Could you check a few things on this model? Use its own coordinates, in mm. Coordinates: 2 decimals unless noted, no trailing zeros.
Autodesk Inventor part; units mm, degrees
ref_plane "Work Plane1" through (387.8168, 0.3965, 6.35) normal (0, 0, 1) x (1, 0, 0)
ref_plane "YZ Plane" through (0, 0, 0) normal (1, 0, 0) x (0, 1, 0)
ref_plane "XZ Plane" through (0, 0, 0) normal (0, 1, 0) x (-1, 0, 0)
sketch "Sketch1" plane through (0, 0, 0) normal (0, 0, 1) x (1, 0, 0)
  line L0 (-374.9457, 6.7465) -> (391.8168, 6.7465)
  line L1 (391.8168, 6.7465) -> (391.8168, -5.9535)
  line L2 (391.8168, -5.9535) -> (-374.9457, -5.9535)
  line L3 (-374.9457, -5.9535) -> (-374.9457, 6.7465)
  dimension "d0" = 766.7625
  dimension "d1" = 12.7
extrude "Extrusion1" add sketch "Sketch1" along normal blind 12.7
hole "Hole3" at (-358.4357, 0.3965, 12.7) direction (0, 0, -1) diameter 5 end through all
hole "Hole4" at (-320.3357, 0.3965, 12.7) direction (0, 0, -1) diameter 5 end through all
hole "Hole5" at (-244.2881, 0.3965, 12.7) direction (0, 0, -1) diameter 5 end through all
hole "Hole6" at (-117.2881, 0.3965, 12.7) direction (0, 0, -1) diameter 5 end through all
hole "Hole7" at (9.7119, 0.3965, 12.7) direction (0, 0, -1) diameter 5 end through all
hole "Hole8" at (136.7119, 0.3965, 12.7) direction (0, 0, -1) diameter 5 end through all
hole "Hole9" at (263.7119, 0.3965, 12.7) direction (0, 0, -1) diameter 5 end through all
hole "Hole10" at (281.7967, 0.3965, 12.7) direction (0, 0, -1) diameter 5 end through all
hole "Hole11" at (307.1967, 0.3965, 12.7) direction (0, 0, -1) diameter 5 end through all
hole "Hole12" at (391.8168, 0.3965, 6.35) direction (-1, 0, 0) diameter 3 depth 8 tip angle 118
ref_plane "Work Plane1" through (387.8168, 0.3965, 6.35) normal (0, 0, 1) x (1, 0, 0)
sketch "Sketch4" plane through (387.8168, 0.3965, 6.35) normal (0, 0, 1) x (1, 0, 0)
  line L0 (4, 6.35) -> (4, -6.35)
  line L1 (4, 0) -> (-4.9613, 0)
  line L2 (-839.4388, 0) -> (234.0288, 0)
  line L3 (4, 2.0193) -> (4, 6.35)
  line L4 (-5.6322, 6.35) -> (4, 2.0193)
  line L5 (-5.6322, 9.0208) -> (4, 9.0208)
  line L6 (4, 9.0208) -> (4, 6.0715)
  line L7 (-5.6322, 6.35) -> (-11.5724, 9.0208)
  line L8 (-5.9043, 9.0208) -> (-11.5724, 9.0208)
  line L9 (-5.6322, 9.0208) -> (-5.9043, 9.0208)
revolve "Revolution2" cut sketch "Sketch4" angle 360 about axis through (391.8168, 0.3965, 6.35) along (-1, 0, 0)
properties part number "Long rod"
(1) We'd pull the mould along Y, two halves only. Please class faces 1 (the face through (-2, 6.746, 6)), 2 (the face through (-374.946, 0, 6)), 3 (the face through (9, -5.954, 6)): +Y half, -Y half, draft (parallel to the pull), parting line (faces both ways), or undercut.
Answers:
face 1: +Y half
face 2: draft
face 3: -Y half
(2) I need wall thicknesses on probe 1 along X at (y, z) = (-3.5, 6.75); probe 2 along X at (y, z) = (3.25, 10). Which ranges of each line are inside material? Lowest first, please.
Answers:
probe 1: x = -374.95 to 387.6
probe 2: x = -374.95 to 386
(3) Imagine slicing it at A-A, the plane z = 2.25. State how many separate pieces and enclosed holes the cut face has, and give its area (3 significant figures).
Answers:
separate pieces: 1
enclosed holes: 9
area: 9,470 mm2
